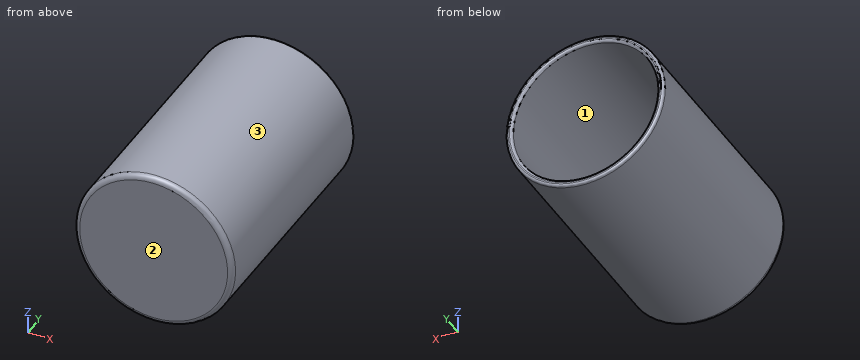
from build123d import *

# Parameters (mm, degrees)
SKETCH1_R           = 38.1
BOSS_EXTRUDE1_DEPTH = 5.08
SKETCH3_R           = 38.1
SKETCH3_R_2         = 34.925
BOSS_EXTRUDE2_DEPTH = 109.22
FILLET1_R           = 1.27
FILLET2_R           = 2.54


with BuildPart() as part:
    # Sketch1 → Boss-Extrude1 (new body)
    with BuildSketch(Plane(origin=(0, 0, 0), x_dir=(1, 0, 0), z_dir=(0, 1, 0))):
        with Locations(Location((0, 0, 0), (0, 0, 270))):
            Circle(SKETCH1_R)
    extrude(amount=BOSS_EXTRUDE1_DEPTH)

    # Sketch3 → Boss-Extrude2 (add)
    with BuildSketch(Plane(origin=(0, 5.08, 0), x_dir=(1, 0, 0), z_dir=(0, 1, 0))):
        with Locations(Location((0, 0, 0), (0, 0, 270))):
            Circle(SKETCH3_R)
        with Locations(Location((0, 0, 0), (0, 0, 270))):
            Circle(SKETCH3_R_2, mode=Mode.SUBTRACT)
    extrude(amount=BOSS_EXTRUDE2_DEPTH)

    # Fillet1
    fillet1_edges = [part.edges().sort_by_distance(p)[0] for p in [
        (0, 114.3, -38.1),
        (0, 114.3, -34.925),
    ]]
    fillet(fillet1_edges, radius=FILLET1_R)

    # Fillet2
    fillet2_edges = [part.edges().sort_by_distance(p)[0] for p in [
        (0, 0, -38.1),
    ]]
    fillet(fillet2_edges, radius=FILLET2_R)


solid = part.part
Input: part model. Units: mm. Frame: model coordinates. Face numbers are marked on the shaded views. Give positions to 0.01 mm unless a question says otherwise; leave off trailing zeros. Loops run counter-clockwise (first coordinate to the right, second up) from the corner with the lowest first, then second, coordinate; pieces in that order, holes last. Notation, with made-up numbers: M 28,-27.5 L 43,-27.5 A35 ccw 43,6.5 Z; hole C 36,-19.75 d2. An arc over 180 degrees is marked long. Use CSV: the item, a comma, the result in double quotes.
(1) Pull-direction query (X, two-part tool) for the marked faces 1, 2 and 3; classes: pulls with the +X half, pulls with the -X half, needs draft (parallel to the pull), parting line crosses it, or undercut.
Outcome:
face 1,"undercut"
face 2,"needs draft"
face 3,"parting line crosses it"
(2) Material intervals for L1, parallel to X at y = 53, z = 0 (3 decimals); L2, parallel to Z at x = 15.5, y = 57.5; L3, parallel to Y at x = -6.5, z = 26, sorted ascending. Write a range as [from, to].
Outcome:
L1,"x = [-38.1, -34.925], [34.925, 38.1]"
L2,"z = [-34.8, -31.3], [31.3, 34.8]"
L3,"y = [0, 5.08]"
(3) Section A-A, the plane x = 0. Return loops of the section in (y, z) (3 decimals).
Outcome:
outline,"M 0,-35.56 A2.54 ccw 2.54,-38.1 L 113.03,-38.1 A1.27 ccw 114.3,-36.83 L 114.3,-36.195 A1.27 ccw 113.03,-34.925 L 5.08,-34.925 L 5.08,34.925 L 113.03,34.925 A1.27 ccw 114.3,36.195 L 114.3,36.83 A1.27 ccw 113.03,38.1 L 2.54,38.1 A2.54 ccw 0,35.56 Z"
(4) Pin query (flat end, axial travel): P1, Ø10, axis at x = 25.5, y = 64, coming from the +Z side; P2, Ø1, axis at y = 97.5, z = 29, coming from the -X side; P3, Ø4, axis at y = 18.5, z = 4.5, coming from the -X side. Return the tip coordinate at first contact, or that it passes through.
Outcome:
P1,"stops at z = 32.11"
P2,"stops at x = -25.29"
P3,"stops at x = -38.02"
(5) Section B-B, the plane z = 0. Return loops of the section in (x, y) (3 decimals), plus the area to 3 significant figures.
Outcome:
outline,"M -38.1,2.54 A2.54 ccw -35.56,0 L 35.56,0 A2.54 ccw 38.1,2.54 L 38.1,113.03 A1.27 ccw 36.83,114.3 L 36.195,114.3 A1.27 ccw 34.925,113.03 L 34.925,5.08 L -34.925,5.08 L -34.925,113.03 A1.27 ccw -36.195,114.3 L -36.83,114.3 A1.27 ccw -38.1,113.03 Z"
area,"1,080 mm²"
(6) Section C-C, the plane y = 73.5. Return loops of the section in (x, z) (3 decimals), plus the area to 3 significant figures.
Outcome:
outline,"C 0,0 d76.2; hole C 0,0 d69.85"
area,"728 mm²"
